Model file for the job. Use its own axes, mm. Face numbers are marked on the shaded views. A direction names the side the tool comes from. Give positions to 0.01 mm unless a question says otherwise; leave off trailing zeros. Write each loop counter-clockwise with the first axis right and the second up, starting at its lowest first coordinate (ties: lowest second). Pieces come first, ordered by that corner, then holes. Notation, with made-up numbers: (35, 76) - (77, 76) arc R24 cw to (77, 91) - close; hole circle Ø4 at (85, 75.5). An arc over 180 degrees is marked (long way). Use a Markdown table: item, result. Add a question column.
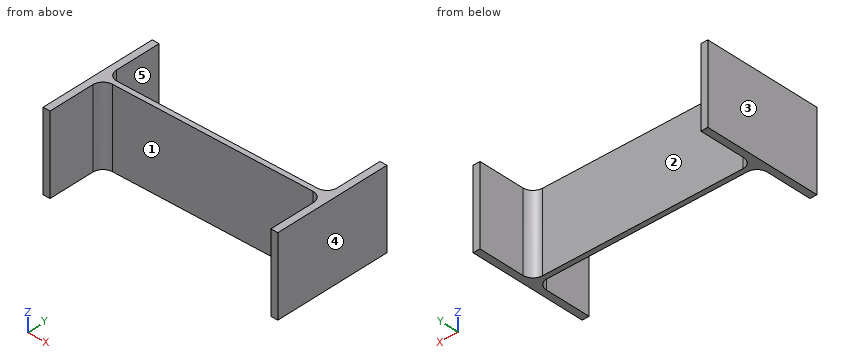
Autodesk Fusion 360 part; units mm, degrees
sketch "スケッチ1" plane through (0, 0, 0) normal (0, 0, 1) x (1, 0, 0)
  line L0 (0, 75) -> (0, -75)
  line L1 (300, -75) -> (300, 75)
  line L2 (291, -16.25) -> (291, -75)
  line L3 (9, -75) -> (9, -16.25)
  line L4 (0, -75) -> (9, -75)
  line L5 (291, -75) -> (300, -75)
  line L6 (278, 3.25) -> (22, 3.25)
  line L7 (22, -3.25) -> (278, -3.25)
  line L8 (9, 16.25) -> (9, 75)
  arc A0 (22, -3.25) -> (9, -16.25) centre (22, -16.25) ccw
  arc A1 (9, 16.25) -> (22, 3.25) centre (22, 16.25) ccw
  line L9 (9, 75) -> (0, 75)
  line L10 (291, 75) -> (291, 16.25)
  arc A2 (291, -16.25) -> (278, -3.25) centre (278, -16.25) ccw
  arc A3 (278, 3.25) -> (291, 16.25) centre (278, 16.25) ccw
  line L11 (300, 75) -> (291, 75)
extrude "押し出し1" add sketch "スケッチ1" along normal blind 100
(1) Flat gauge pins, fed straight in: pin 1 (12 mm diameter, centred on x = 132, y = -15, fed in from -Z); pin 2 (4 mm diameter, centred on x = 257.5, z = 22, fed in from -Y). Where does each tip first touch, or does it go through?
(2) Band-saw the part on A-A (y = -44). Write the cut outline in (x, z).
(3) Probe probe 1 along X at (y, z) = (40, 37); probe 2 along Y at (x, z) = (82, 26); probe 3 along X at (y, z) = (9.5, 10). List the from-to ranges inside material, lowest first. Write a range as [from, to].
(4) Band-saw the part on D-D (y = 8). Write the cut outline in (x, z), then the cut area to 3 significant figures.
(5) Which spindle directions (+Z, -Z, +X, -X, +Y, -Y) get a long thin tool onto all of the face, cutting with end or side? Do the marked faces 1 and 2. Say none if no direction does.
(6) Two-plate mould, pull along X, no slides. Class the marked faces 3, 4 and 5: +X half, -X half, draft (parallel to the pull), parting line (faces both ways), or undercut.
(7) Band-saw the part on B-B (z = 12). Write the cut outline in (x, y), then the cut area to 3 significant figures.
(8) Band-saw the part on C-C (x = 204.5). Write the cut outline in (y, z), then the cut area to 3 significant figures.
Model answer:
| question | item | result |
|---|---|---|
| 1 | pin 1 | passes through |
| 1 | pin 2 | stops at y = -3.25 |
| 2 | outline | (0, 0) - (9, 0) - (9, 100) - (0, 100) - close; (291, 0) - (300, 0) - (300, 100) - (291, 100) - close |
| 3 | probe 1 | x = [0, 9], [291, 300] |
| 3 | probe 2 | y = [-3.25, 3.25] |
| 3 | probe 3 | x = [0, 10.89], [289.11, 300] |
| 4 | outline | (0, 0) - (11.95, 0) - (11.95, 100) - (0, 100) - close; (288.05, 0) - (300, 0) - (300, 100) - (288.05, 100) - close |
| 4 | area | 2,390 mm^2 |
| 5 | face 1 | +Z, -Z, -Y |
| 5 | face 2 | +Z, -Z, +Y |
| 6 | face 3 | -X half |
| 6 | face 4 | +X half |
| 6 | face 5 | undercut |
| 7 | outline | (0, -75) - (9, -75) - (9, -16.25) arc R13 cw to (22, -3.25) - (278, -3.25) arc R13 cw to (291, -16.25) - (291, -75) - (300, -75) - (300, 75) - (291, 75) - (291, 16.25) arc R13 cw to (278, 3.25) - (22, 3.25) arc R13 cw to (9, 16.25) - (9, 75) - (0, 75) - close |
| 7 | area | 4,680 mm^2 |
| 8 | outline | (-3.25, 0) - (3.25, 0) - (3.25, 100) - (-3.25, 100) - close |
| 8 | area | 650 mm^2 |
